```python
from build123d import *

# Parameters (mm, degrees)
BOSS_EXTRUDE1_DEPTH = 25
CUT_EXTRUDE2_DEPTH  = 59.736700622
SKETCH4_W           = 10
SKETCH4_H           = 40
CUT_EXTRUDE3_DEPTH  = 57.5
CUT_EXTRUDE4_DEPTH  = 1
SKETCH6_R           = 5
CUT_EXTRUDE5_DEPTH  = 44.011626335
SKETCH9_W           = 3.25
SKETCH9_H           = 40
CUT_EXTRUDE6_DEPTH  = 77.974021592


with BuildPart() as part:
    # Sketch1 → Boss-Extrude1 (new body)
    with BuildSketch(Plane.XY):
        with BuildLine():
            Line((-35, -14), (-35, 14))
            ThreePointArc((-35, 14), (-33.242640687, 18.242640687), (-29, 20))
            Line((-29, 20), (8.634575376, 20))
            ThreePointArc((8.634575376, 20), (9.965959981, 19.850420073), (11.230961782, 19.409138345))
            Line((11.230961782, 19.409138345), (30.461848541, 10.1783127))
            ThreePointArc((30.461848541, 10.1783127), (33.771070385, 7.22671574), (35, 2.966128241))
            Line((35, 2.966128241), (35, -2.966128241))
            ThreePointArc((35, -2.966128241), (33.771070385, -7.22671574), (30.461848541, -10.1783127))
            Line((30.461848541, -10.1783127), (11.230961782, -19.409138345))
            ThreePointArc((11.230961782, -19.409138345), (9.965959981, -19.850420073), (8.634575376, -20))
            Line((8.634575376, -20), (-29, -20))
            ThreePointArc((-29, -20), (-33.242640687, -18.242640687), (-35, -14))
        make_face()
    extrude(amount=BOSS_EXTRUDE1_DEPTH)

    # Sketch3 → Cut-Extrude2 (cut, through all)
    with BuildSketch(Plane(origin=(0, -20, 0), x_dir=(-1, 0, 0), z_dir=(0, -1, 0))):
        with BuildLine():
            Line((-0.88003088, -25), (24.11996912, -25))
            ThreePointArc((24.11996912, -25), (11.61996912, -12.5), (-0.88003088, -25))
        make_face()
        Polygon((11.619969205, -10), (29, -10), (29, 0), (-8.634575376, 0), (-8.634575376, -10), align=None)
    extrude(amount=-CUT_EXTRUDE2_DEPTH, mode=Mode.SUBTRACT)

    # Sketch4 → Cut-Extrude3 (cut, symmetric)
    with BuildSketch(Plane.ZY.offset(-8.634575376)):
        with Locations((5, 0)):
            Rectangle(SKETCH4_W, SKETCH4_H)
    extrude(amount=CUT_EXTRUDE3_DEPTH, both=True, mode=Mode.SUBTRACT)

    # Sketch5 → Cut-Extrude4 (cut)
    with BuildSketch(Plane(origin=(0, 0, 10), x_dir=(-1, 0, 0), z_dir=(0, 0, -1))):
        with BuildLine():
            Line((-2.634575376, -14), (26, -14))
            ThreePointArc((26, -14), (28.121320344, -13.121320344), (29, -11))
            Line((29, -11), (29, 11))
            ThreePointArc((29, 11), (28.121320344, 13.121320344), (26, 14))
            Line((26, 14), (-2.634575376, 14))
            ThreePointArc((-2.634575376, 14), (-4.75589572, 13.121320344), (-5.634575376, 11))
            Line((-5.634575376, 11), (-5.634575376, -11))
            ThreePointArc((-5.634575376, -11), (-4.75589572, -13.121320344), (-2.634575376, -14))
        make_face()
    extrude(amount=-CUT_EXTRUDE4_DEPTH, mode=Mode.SUBTRACT)

    # Sketch6 → Cut-Extrude5 (cut, through all)
    with BuildSketch(Plane(origin=(0, 0, 10), x_dir=(-1, 0, 0), z_dir=(0, 0, -1))):
        with Locations((-19.280961782, 0)):
            Circle(SKETCH6_R)
    extrude(amount=-CUT_EXTRUDE5_DEPTH, mode=Mode.SUBTRACT)

    # Sketch9 → Cut-Extrude6 (cut, through all)
    with BuildSketch(Plane.ZY.offset(35)):
        with Locations((23.375, 0)):
            Rectangle(SKETCH9_W, SKETCH9_H)
    extrude(amount=-CUT_EXTRUDE6_DEPTH, mode=Mode.SUBTRACT)


solid = part.part
```
CAD build for the part. Positions are in the model's coordinates, mm. A direction names the side the tool comes from. Round coordinates to 2 decimals unless told otherwise and drop trailing zeros. Loops run counter-clockwise (first coordinate to the right, second up) from the corner with the lowest first, then second, coordinate; pieces in that order, holes last. Notation, with made-up numbers: (-25.5, 73.25) - (22.5, 73.25) arc R27 ccw to (22.5, 94.25) - close; hole circle Ø4 at (18.25, 34). An arc over 180 degrees is marked (long way). Return JSON: item names as keys, results as strings. Group by question number.
Q1. Band-saw the part on C-C on y = 0. Give the cut face in (x, z), plus the area to 3 significant figures.
Q2. Band-saw the part on A-A on z = 13.25. Give the cut face in (x, y).
Q3. Band-saw the part on D-D on z = 19. Give the cut face in (x, y), plus the area to 3 significant figures.
Q4. Tool access for faces 1 (the face through (14, 0, 21.75)), 2 (the face through (4.732, 13.145, 10.493)): list every direction of +Z, -Z, +X, -X, +Y, -Y with a clear straight run to the whole face (end or side of a thin tool).
Q5. Two-plate mould, pull along Y, no slides. Class faces 3 (the face through (20.98, -14.73, 15.79)), 4 (the face through (-29, 0, 21.75)), 5 (the face through (-10, 20, 12)), 6 (the face through (-11, 0, 11)): +Y half, -Y half, draft (parallel to the pull), parting line (faces both ways), or undercut.
Q6. Flat gauge pin, fed straight in: pin 1 Ø1 at (x, y) = (-24, 5) entering from -Z. Where does the tip first touch, or does it go through?
Q7. Band-saw the part on B-B on x = -24.5. Give the cut face in (y, z), plus the area to 3 significant figures.
Q8. Drill centre lines: line 1 along Z through (x, y) = (3.5, -1); line 2 along X through (y, z) = (-7.5, 15.75); line 3 along Y through (x, z) = (23.5, 19.75). Where is each one in solid material? Low to high. Write a range as [from, to].
Solutions:
{
 "1": {"outline": "(-35, 10) - (-29, 10) - (-29, 11) - (5.63, 11) - (5.63, 10) - (14.28, 10) - (14.28, 21.75) - (0.45, 21.75) arc R12.5 cw to (-23.69, 21.75) - (-35, 21.75) - close; (24.28, 10) - (35, 10) - (35, 21.75) - (24.28, 21.75) - close", "area": "505 mm^2"},
 "2": {"outline": "(-35, -14) arc R6 ccw to (-29, -20) - (-15.88, -20) - (-15.88, 20) - (-29, 20) arc R6 ccw to (-35, 14) - close; (-7.36, -20) - (8.63, -20) arc R6 ccw to (11.23, -19.41) - (30.46, -10.18) arc R8 ccw to (35, -2.97) - (35, 2.97) arc R8 ccw to (30.46, 10.18) - (11.23, 19.41) arc R6 ccw to (8.63, 20) - (-7.36, 20) - close; hole circle Ø10 at (19.28, 0)"},
 "3": {"outline": "(-35, -14) arc R6 ccw to (-29, -20) - (-22.59, -20) - (-22.59, 20) - (-29, 20) arc R6 ccw to (-35, 14) - close; (-0.65, -20) - (8.63, -20) arc R6 ccw to (11.23, -19.41) - (30.46, -10.18) arc R8 ccw to (35, -2.97) - (35, 2.97) arc R8 ccw to (30.46, 10.18) - (11.23, 19.41) arc R6 ccw to (8.63, 20) - (-0.65, 20) - close; hole circle Ø10 at (19.28, 0)", "area": "1,520 mm^2"},
 "4": {"face 1": "+Z, +X, -X, +Y, -Y", "face 2": "-Z"},
 "5": {"face 3": "-Y half", "face 4": "draft", "face 5": "+Y half", "face 6": "undercut"},
 "6": {"pin 1": "stops at z = 11"},
 "7": {"outline": "(-20, 10) - (-14, 10) - (-14, 11) - (14, 11) - (14, 10) - (20, 10) - (20, 21.75) - (-20, 21.75) - close", "area": "442 mm^2"},
 "8": {"line 1": "z = [11, 21.75]", "line 2": "x = [-35, -20.03], [-3.21, 33.59]", "line 3": "y = [-13.52, -2.68], [2.68, 13.52]"}
}
